Autodesk Inventor part; units mm, degrees
ref_plane "Start plane" through (0, 0, 0) normal (0, 0, 1) x (1, 0, 0)
ref_plane "End plane" through (0, 0, 707.1068) normal (0, 0, 1) x (1, 0, 0)
ref_plane "Work Plane4" through (1691.7009, -22, 2368.8077) normal (-0.7071, 0, 0.7071) x (0.7071, 0, 0.7071)
ref_plane "Start plane" through (0, 0, 0) normal (0, 0, 1) x (1, 0, 0)
ref_plane "End plane" through (0, 0, 707.1068) normal (0, 0, 1) x (1, 0, 0)
sketch "Sketch" plane through (0, 0, 0) normal (0, 0, 1) x (1, 0, 0)
  line L0 (-30, -24) -> (-30, 24)
  line L1 (-24, 30) -> (24, 30)
  line L2 (30, 24) -> (30, -24)
  line L3 (24, -30) -> (-24, -30)
  arc A0 (-30, -24) -> (-24, -30) centre (-24, -24) ccw
  arc A1 (30, 24) -> (24, 30) centre (24, 24) ccw
  arc A2 (-24, 30) -> (-30, 24) centre (-24, 24) ccw
  arc A3 (24, -30) -> (30, -24) centre (24, -24) ccw
  arc A4 (-24, 27) -> (-27, 24) centre (-24, 24) ccw
  line L4 (-24, 27) -> (24, 27)
  arc A5 (27, 24) -> (24, 27) centre (24, 24) ccw
  line L5 (27, 24) -> (27, -24)
  arc A6 (24, -27) -> (27, -24) centre (24, -24) ccw
  line L6 (24, -27) -> (-24, -27)
  arc A7 (-27, -24) -> (-24, -27) centre (-24, -24) ccw
  line L7 (-27, -24) -> (-27, 24)
  line L8 (0, 43.7397) -> (0, -43.7397) construction
  line L9 (-43.7397, 0) -> (43.7397, 0) construction
  dimension "d7" = 6
  dimension "d9" = 60
  dimension "d11" = 60
  dimension "d12" = 3
  dimension "d15" = 30
  dimension "d16" = 30
extrude "Body" add sketch "Sketch" along normal up to surface (707.1068 mm away) from surface at 0
sketch "Sketch3" plane through (0, 0, 0) normal (0, 0, 1) x (1, 0, 0)
  line L0 (0, 0) -> (10, 0)
ref_plane "Work Plane3" through (0, 0, 0) normal (0, -1, 0) x (1, 0, 0)
ref_plane "Work Plane4" through (1691.7009, -22, 2368.8077) normal (-0.7071, 0, 0.7071) x (0.7071, 0, 0.7071)
split "Split1" plane through (1691.7009, -22, 2368.8077) removes the side toward (-0.7071, 0, 0.7071)
ref_plane "Work Plane5" through (-323.5534, 50, 353.5534) normal (-0.7071, 0, -0.7071) x (-0.7071, 0, 0.7071)
split "Split2" plane through (-323.5534, 50, 353.5534) removes the side toward (-0.7071, 0, -0.7071)
sketch "Sketch4" plane through (0, 0, 0) normal (0, -1, 0) x (1, 0, 0)
  line L0 (-2, 0) -> (12, 0)
  line L1 (-2, 707.1068) -> (12, 707.1068)
  dimension "d18" = 707.1068
equation "\"d7\" = G_IR"
equation "\"d9\" = G_W"
equation "\"d11\" = G_H"
equation "\"d12\" = G_T"
equation "\"d15\" = 0.5 * d9"
equation "\"d16\" = 0.5 * d11"
equation "\"d3\" = G_L"
equation "\"G_W\" = 60"
equation "\"G_H\" = 60"
equation "\"G_T\" = 3"
equation "\"G_IR\" = 6"
equation "\"G_L\" = d18"
equation "\"G_OFFSET_START\" = 0"
equation "\"G_OFFSET_END\" = -141.42136"
equation "\"d14\" = G_OFFSET_END + B_L"
equation "\"B_L\" = 848.52814"
properties part number "ISO 10799-2 - 60x60x3 - 707,11" material "Steel, Mild"
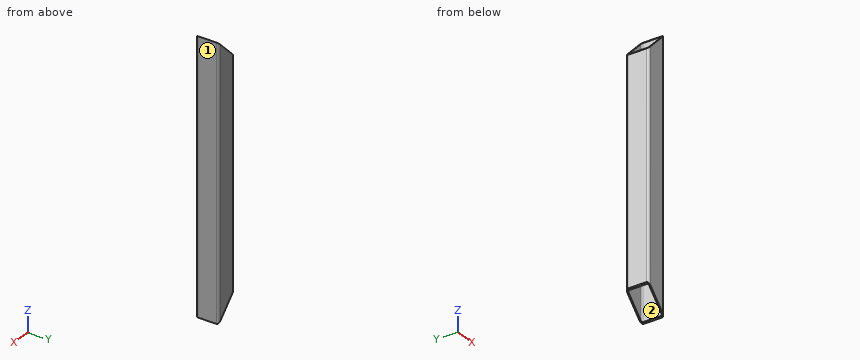
Input: part model. Units: mm. Frame: model coordinates. Face numbers are marked on the shaded views. Coordinates: 2 decimals unless noted, no trailing zeros. Order: outer loops, then holes, each group sorted by start corner. A loop starts at its lowest first (then second) coordinate and runs counter-clockwise, first axis right, second up. Notation, with made-up numbers: (64.25, 19.25) - (119.25, 19.25) arc R23 cw to (119.25, 42.25) - close; hole circle Ø3 at (8.25, -36.5). An arc over 180 degrees is marked (long way). Return JSON: item names as keys, results as strings.
Q1. Cut plane B-B (y = 12). Return loops of the section in (x, z), then the cut area to 3 significant figures.
The answers:
{"outline": "(-30, 60) - (-27, 57) - (-27, 650.11) - (-30, 647.11) - close; (27, 3) - (30, 0) - (30, 707.11) - (27, 704.11) - close", "area": "3,880 mm2"}
Q2. Ray query, probe 1 along X at (y, z) = (-13, 192); probe 2 along Y at (x, z) = (25, 417.5). Return the intervals inside material, ascending.
The answers:
{"probe 1": "x = -30 to -27, 27 to 30", "probe 2": "y = -29.92 to -26.83, 26.83 to 29.92"}
Q3. Draft query along Y for the marked faces 1 and 2. Return one class per face: +Y half, -Y half, draft (parallel to the pull), parting line (faces both ways), or undercut.
The answers:
{"face 1": "draft", "face 2": "undercut"}
Q4. Cut plane A-A (z = 354). Return loops of the section in (x, y).
The answers:
{"outline": "(-30, -24) arc R6 ccw to (-24, -30) - (24, -30) arc R6 ccw to (30, -24) - (30, 24) arc R6 ccw to (24, 30) - (-24, 30) arc R6 ccw to (-30, 24) - close; hole (-27, -24) arc R3 ccw to (-24, -27) - (24, -27) arc R3 ccw to (27, -24) - (27, 24) arc R3 ccw to (24, 27) - (-24, 27) arc R3 ccw to (-27, 24) - close"}
Q5. Cut plane C-C (x = 7.5). Return loops of the section in (y, z).
The answers:
{"outline": "(-30, 22.5) - (-27, 22.5) - (-27, 684.61) - (-30, 684.61) - close; (27, 22.5) - (30, 22.5) - (30, 684.61) - (27, 684.61) - close"}
